Here's the drawing with two shaded views (mm, measured from the low corner). I have some questions. A direction names the side the tool comes from. Round coordinates to 2 decimals unless told otherwise and drop trailing zeros. Loops run counter-clockwise (first coordinate to the right, second up) from the corner with the lowest first, then second, coordinate; pieces in that order, holes last.
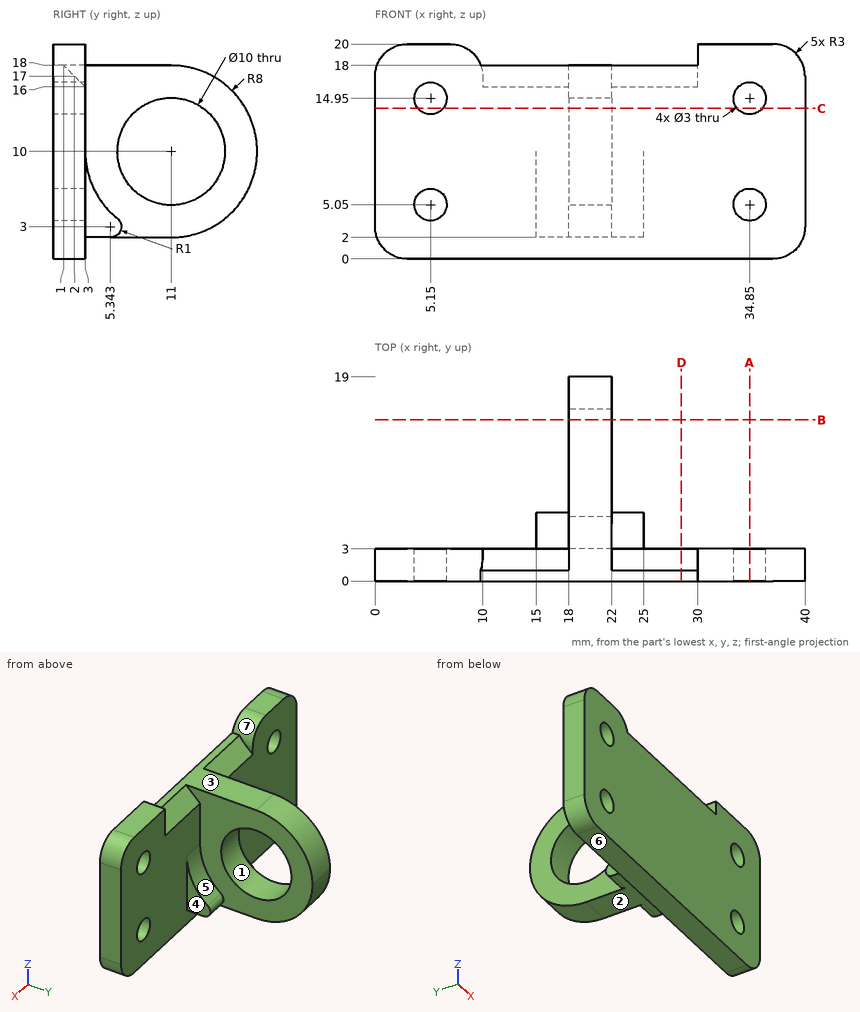
Item 1: If we section it at C-C, the plane z = 14: Please give me the cut outline in (x, y), then the cut area to 3 significant figures.
Results list:
outline: (0, 0) - (3.99, 0) - (3.99, 3) - (0, 3) - close; (6.31, 0) - (33.69, 0) - (33.69, 3) - (22, 3) - (22, 8) - (18, 8) - (18, 3) - (6.31, 3) - close; (18, 14) - (22, 14) - (22, 17.93) - (18, 17.93) - close; (36.01, 0) - (40, 0) - (40, 3) - (36.01, 3) - close
area: 142 mm2
Item 2: If I drill on line 1 along X through (y, z) = (0.9, 14.95); line 2 along X through (y, z) = (16.5, 11); line 3 along Y through (x, z) = (14, 2.25), over which ranges is the centre line in solid material (lowest first)?
Results list:
line 1: x = 0 to 3.65, 6.65 to 33.35, 36.35 to 40
line 2: x = 18 to 22
line 3: y = 0 to 3
Item 3: If we section it at D-D, the plane x = 28.5: Please give me the cut outline in (y, z), then the cut area to 3 significant figures.
Results list:
outline: (0, 0) - (3, 0) - (3, 16) - (1, 18) - (0, 18) - close
area: 52.0 mm2
Item 4: If we section it at A-A, the plane x = 34.85: Please give me the cut outline in (y, z), then the cut area to 3 significant figures.
Results list:
outline: (0, 0) - (3, 0) - (3, 3.55) - (0, 3.55) - close; (0, 6.55) - (3, 6.55) - (3, 13.45) - (0, 13.45) - close; (0, 16.45) - (3, 16.45) - (3, 20) - (0, 20) - close
area: 42.0 mm2
Item 5: Will these pins go through, and if not, where does the flat tip stop? pin 1 (1.7 mm diameter, centred on y = 5, z = 7.5, fed in from -X); pin 2 (10 mm diameter, centred on x = 19.5, y = 15.5, fed in from +Z); pin 3 (1.5 mm diameter, centred on y = 16, z = 15, fed in from +X).
Results list:
pin 1: stops at x = 18
pin 2: stops at z = 18
pin 3: stops at x = 22
Item 6: For the marked faces 5, 6 and 7, which set-ups out of +Z, -Z, +X, -X, +Y, -Y let a thin tool reach every point of the face, with its end or its side?
Results list:
face 5: +Z, +X, +Y
face 6: -Z, +X, -X, +Y, -Y
face 7: +Z, +Y
Item 7: If we section it at B-B, the plane y = 15: Please give me the cut outline in (x, z).
Results list:
outline: (18, 3.07) - (22, 3.07) - (22, 7) - (18, 7) - close; (18, 13) - (22, 13) - (22, 16.93) - (18, 16.93) - close
Item 8: We'd pull the mould along Z, two halves only. Please class the marked faces 1, 2, 3 and 4: released by +Z, released by -Z, zero draft, split by the parting line, or undercut.
Results list:
face 1: undercut
face 2: released by -Z
face 3: released by +Z
face 4: zero draft
